Source: CAD feature listing. Evaluate the final solid. Frame: model axes, mm. Round coordinates to 2 decimals unless told otherwise and drop trailing zeros. Order: outer loops, then holes, each group sorted by start corner. A loop starts at its lowest first (then second) coordinate and runs counter-clockwise, first axis right, second up. Notation, with made-up numbers: M 23,53 L 44,53 A36 cw 44,87 Z; hole C 66.25,13.25 d6. An arc over 180 degrees is marked long. Use one line per item in the form item = value. Start each with the question number.
Q1. Section C-C (z = -2.5). Return the cut outline in (x, y).
Q2. Section D-D (y = 2.95). Give the number of separate pieces and of enclosed holes in the cut face, plus the area to 3 significant figures.
Q3. Section A-A (z = 39). Return the cut outline in (x, y), plus the area to 3 significant figures.
Q4. Section B-B (x = -15.5). Return the cut outline in (y, z).
Q5. Material intervals for probe 1 along X at (y, z) = (4.1, -76); probe 2 along X at (y, z) = (0.55, 12); probe 3 along X at (y, z) = (0.25, 49.5), sorted ascending.
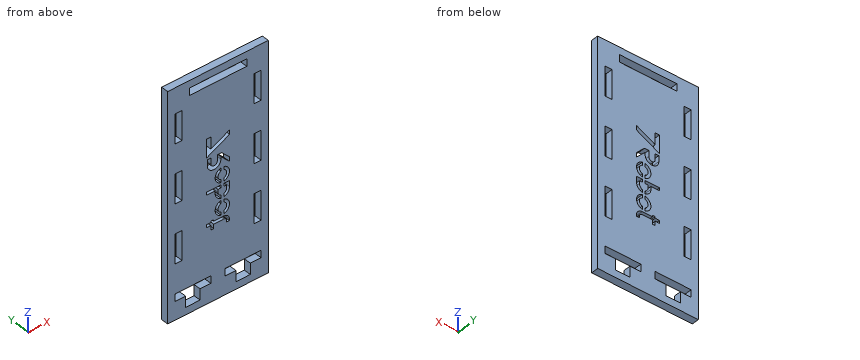
from build123d import *

# Parameters (mm, degrees)
ESQUISSE1_W             = 70
ESQUISSE1_H             = 155
ESQUISSE1_W_2           = 5
ESQUISSE1_H_2           = 20
ESQUISSE1_W_3           = 40
ESQUISSE1_H_3           = 5
BOSS_EXTRU_1_DEPTH      = 5
ENL_V_MAT_EXTRU_1_DEPTH = 5


with BuildPart() as part:
    # Esquisse1 → Boss.-Extru.1 (new body)
    with BuildSketch(Plane(origin=(0, 0, 0), x_dir=(1, 0, 0), z_dir=(0, 1, 0))):
        with Locations((0, 5)):
            Rectangle(ESQUISSE1_W, ESQUISSE1_H)
        Polygon((-22.5, 77.5), (-12.5, 77.5), (-12.5, 70), (-5, 70), (-5, 65), (-30, 65), (-30, 70), (-22.5, 70), align=None, mode=Mode.SUBTRACT)
        with Locations((27.5, 35)):
            Rectangle(ESQUISSE1_W_2, ESQUISSE1_H_2, mode=Mode.SUBTRACT)
        with Locations((-27.5, 35)):
            Rectangle(ESQUISSE1_W_2, ESQUISSE1_H_2, mode=Mode.SUBTRACT)
        Polygon((12.5, 77.5), (22.5, 77.5), (22.5, 70), (30, 70), (30, 65), (5, 65), (5, 70), (12.5, 70), align=None, mode=Mode.SUBTRACT)
        with Locations((-27.5, -5)):
            Rectangle(ESQUISSE1_W_2, ESQUISSE1_H_2, mode=Mode.SUBTRACT)
        with Locations((-27.5, -45)):
            Rectangle(ESQUISSE1_W_2, ESQUISSE1_H_2, mode=Mode.SUBTRACT)
        with Locations((27.5, -5)):
            Rectangle(ESQUISSE1_W_2, ESQUISSE1_H_2, mode=Mode.SUBTRACT)
        with Locations((27.5, -45)):
            Rectangle(ESQUISSE1_W_2, ESQUISSE1_H_2, mode=Mode.SUBTRACT)
        with Locations((0, -65)):
            Rectangle(ESQUISSE1_W_3, ESQUISSE1_H_3, mode=Mode.SUBTRACT)
    extrude(amount=BOSS_EXTRU_1_DEPTH)

    # Esquisse2 → Enlèv. mat.-Extru.1 (cut)
    with BuildSketch(Plane(origin=(0, 5, 0), x_dir=(1, 0, 0), z_dir=(0, 1, 0))):
        Polygon((-8, -27.5), (-5, -27.5), (-5, -19.5), (8, -26), (8, -23), (-8, -15), align=None)
        with BuildLine():
            Line((8, -5), (8, -8))
            Line((8, -8), (2.5, -13.5))
            Line((2.5, -13.5), (-0.5, -13.5))
            Line((-0.5, -13.5), (-0.5, -9.5))
            ThreePointArc((-0.5, -9.5), (-2.75, -7.25), (-5, -9.5))
            Line((-5, -9.5), (-5, -13.5))
            Line((-5, -13.5), (-7.5, -13.5))
            Line((-7.5, -13.5), (-7.5, -9.5))
            ThreePointArc((-7.5, -9.5), (-2.75, -4.75), (2, -9.5))
            Line((2, -9.5), (2, -11))
            Line((2, -11), (8, -5))
        make_face()
        with BuildLine():
            Line((2, -3.5), (2, -1.429447639))
            ThreePointArc((2, -1.429447639), (0, 1.398979486), (2, 4.22740661))
            Line((2, 4.22740661), (2, 6.297958971))
            ThreePointArc((2, 6.297958971), (-2, 1.398979486), (2, -3.5))
        make_face()
        with BuildLine():
            Line((4, 6.297958971), (4, 4.22740661))
            ThreePointArc((4, 4.22740661), (6, 1.398979486), (4, -1.429447639))
            Line((4, -1.429447639), (4, -3.5))
            ThreePointArc((4, -3.5), (8, 1.398979486), (4, 6.297958971))
        make_face()
        with BuildLine():
            Line((-8, 7.797958971), (2, 7.797958971))
            Line((2, 7.797958971), (2, 9.797958971))
            Line((2, 9.797958971), (0, 9.797958971))
            Line((0, 9.797958971), (0, 11.797958971))
            ThreePointArc((0, 11.797958971), (0.550510257, 13.530009779), (2, 14.626386096))
            Line((2, 14.626386096), (2, 16.696938457))
            ThreePointArc((2, 16.696938457), (-0.872983346, 14.960236631), (-2, 11.797958971))
            Line((-2, 11.797958971), (-2, 9.797958971))
            Line((-2, 9.797958971), (-8, 9.797958971))
            Line((-8, 9.797958971), (-8, 7.797958971))
        make_face()
        with BuildLine():
            Line((4, 7.797958971), (8, 7.797958971))
            Line((8, 7.797958971), (8, 11.797958971))
            ThreePointArc((8, 11.797958971), (6.872983346, 14.960236631), (4, 16.696938457))
            Line((4, 16.696938457), (4, 14.626386096))
            ThreePointArc((4, 14.626386096), (5.449489743, 13.530009779), (6, 11.797958971))
            Line((6, 11.797958971), (6, 9.797958971))
            Line((6, 9.797958971), (4, 9.797958971))
            Line((4, 9.797958971), (4, 7.797958971))
        make_face()
        with BuildLine():
            Line((2, 18.196938457), (2, 20.267490818))
            ThreePointArc((2, 20.267490818), (0, 23.095917942), (2, 25.924345067))
            Line((2, 25.924345067), (2, 27.994897428))
            ThreePointArc((2, 27.994897428), (-2, 23.095917942), (2, 18.196938457))
        make_face()
        with BuildLine():
            Line((4, 27.994897428), (4, 25.924345067))
            ThreePointArc((4, 25.924345067), (6, 23.095917942), (4, 20.267490818))
            Line((4, 20.267490818), (4, 18.196938457))
            ThreePointArc((4, 18.196938457), (8, 23.095917942), (4, 27.994897428))
        make_face()
        with BuildLine():
            Line((-8, 29.494897428), (-5, 29.494897428))
            Line((-5, 29.494897428), (-5, 28.494897428))
            Line((-5, 28.494897428), (-3, 28.494897428))
            Line((-3, 28.494897428), (-3, 29.494897428))
            Line((-3, 29.494897428), (4, 29.494897428))
            ThreePointArc((4, 29.494897428), (6.828427125, 30.666470303), (8, 33.494897428))
            Line((8, 33.494897428), (8, 34.494897428))
            Line((8, 34.494897428), (6, 34.494897428))
            Line((6, 34.494897428), (6, 33.494897428))
            ThreePointArc((6, 33.494897428), (5.414213562, 32.080683865), (4, 31.494897428))
            Line((4, 31.494897428), (-3, 31.494897428))
            Line((-3, 31.494897428), (-3, 34.494897428))
            Line((-3, 34.494897428), (-5, 34.494897428))
            Line((-5, 34.494897428), (-5, 31.494897428))
            Line((-5, 31.494897428), (-8, 31.494897428))
            Line((-8, 31.494897428), (-8, 29.494897428))
        make_face()
    extrude(amount=-ENL_V_MAT_EXTRU_1_DEPTH, mode=Mode.SUBTRACT)


solid = part.part
Results list:
q1.outline = M -35,0 L -30,0 L -30,5 L -35,5 Z; M -25,0 L -1.88,0 L -1.88,5 L -25,5 Z; M 0.21,0 L 5.79,0 L 5.79,5 L 0.21,5 Z; M 7.88,0 L 25,0 L 25,5 L 7.88,5 Z; M 30,0 L 35,0 L 35,5 L 30,5 Z
q2.separate_pieces = 1
q2.enclosed_holes = 18
q2.area = 9,330 mm2
q3.outline = M -35,0 L -30,0 L -30,5 L -35,5 Z; M -25,0 L 25,0 L 25,5 L -25,5 Z; M 30,0 L 35,0 L 35,5 L 30,5 Z
q3.area = 300 mm2
q4.outline = M 0,-82.5 L 5,-82.5 L 5,-77.5 L 0,-77.5 Z; M 0,-65 L 5,-65 L 5,62.5 L 0,62.5 Z; M 0,67.5 L 5,67.5 L 5,72.5 L 0,72.5 Z
q5.probe_1 = -35 to -22.5, -12.5 to 12.5, 22.5 to 35
q5.probe_2 = -35 to -30, -25 to -7.5, -5 to -0.5, 4 to 25, 30 to 35
q5.probe_3 = -35 to -30, -25 to 25, 30 to 35
